Read the model definition and answer for the solid it produces. Units are mm, in the model's axes. A direction names the side the tool comes from. Give positions to 0.01 mm unless a question says otherwise; leave off trailing zeros. Order: outer loops, then holes, each group sorted by start corner. A loop starts at its lowest first (then second) coordinate and runs counter-clockwise, first axis right, second up. Notation, with made-up numbers: (14, 55) - (68, 55) arc R33 ccw to (68, 89) - close; hole circle Ø7 at (12.5, 44.5). An arc over 180 degrees is marked (long way). Use a Markdown table: item, result. Add a question column.
1. Which of the six approach directions +Z, -Z, +X, -X, +Y, -Y give full straight-line access (tool end or side, diameter ignored) to faces 4 (the cylindrical face through (-3.233, 1.341, 5.507)), 5 (the cylindrical face through (0.867, 3.905, 2.028)), 6 (the flat face through (0, -3, 5))?
2. For a pull along Z with two mould halves and no side action, classify faces 1 (the flat face through (0, 0, 12)), 2 (the cylindrical face through (1.5, -0.07, 9.04)), 3 (the flat face through (-3, 0, 4)) as released by +Z, released by -Z, zero draft, split by the parting line, or undercut.
3. A cutting plane is placed at C-C on y = -3.25. Determine the outline of the cut face in (x, z), and give its area (3 significant figures).
4. Consider L1, parallel to Z at x = 3.25, y = -0.5; L2, parallel to X at y = 0, z = 10.5; L3, parallel to Z at x = -2, y = 0.25. Determine where each line is inside the solid, lowest interval first.
5. A cutting plane is placed at D-D on z = 2.25. Determine the outline of the cut face in (x, y).
6. A cutting plane is placed at A-A on y = 0. Determine the outline of the cut face in (x, z).
7. Flat-ended cylindrical pins translate along their axes: P1, Ø1, axis at y = 1, z = 8.5, coming from the +X side; P2, Ø2, axis at x = -2.5, z = 6, coming from the +Y side. Find the tip coordinate at first contact, or state that the pin passes through.
Autodesk Inventor part; units mm, degrees
ref_plane "YZ Plane" through (0, 0, 0) normal (1, 0, 0) x (0, 1, 0)
ref_plane "XZ Plane" through (0, 0, 0) normal (0, 1, 0) x (-1, 0, 0)
ref_plane "XY Plane" through (0, 0, 0) normal (0, 0, 1) x (1, 0, 0)
sketch "スケッチ1" plane through (0, 0, 0) normal (0, 1, 0) x (-1, 0, 0)
  line L0 (0, 0) -> (0, 12)
  line L1 (0, 0) -> (4, 0)
  line L2 (4, 0) -> (4, 4)
  line L3 (4, 4) -> (2.6, 4)
  line L4 (2.6, 4) -> (2.6, 5) construction
  line L5 (2.6, 5) -> (3.5, 5)
  line L6 (3.5, 5) -> (3.5, 6)
  line L7 (3.5, 6) -> (1.5, 6)
  line L8 (1.5, 6) -> (1.5, 12)
  line L9 (1.5, 12) -> (0, 12)
  arc A0 (2.6, 5) -> (2.6, 4) centre (2.6, 4.5) ccw
  line L10 (2.6, 4.5) -> (2.1, 4.5) construction
  dimension "d4" = 1
  dimension "d5" = 6
  dimension "d7" = 4
  dimension "d8" = 6
  dimension "d11" = 2.1
  dimension "d12" = 3
  dimension "d13" = 8
  dimension "d14" = 7
revolve "回転1" add sketch "スケッチ1" angle 360 about axis through (0, 0, 0) along (0, 0, 1)
thread "ねじ1"
properties part number "SPNFL-BRN-M3-6" material "ステンレス鋼 AISI 304"
Output values:
| question | item | result |
|---|---|---|
| 1 | face 4 | +Z |
| 1 | face 5 | +Z, -Z |
| 1 | face 6 | none |
| 2 | face 1 | released by +Z |
| 2 | face 2 | zero draft |
| 2 | face 3 | undercut |
| 3 | outline | (-2.33, 0) - (2.33, 0) - (2.33, 4) - (-2.33, 4) - close; (-1.3, 5) - (1.3, 5) - (1.3, 6) - (-1.3, 6) - close |
| 3 | area | 21.3 mm² |
| 4 | L1 | 0 to 4, 5 to 6 |
| 4 | L2 | -1.5 to 1.5 |
| 4 | L3 | 0 to 6 |
| 5 | outline | circle Ø8 at (0, 0) |
| 6 | outline | (-4, 0) - (4, 0) - (4, 4) - (2.6, 4) arc R0.5 cw to (2.6, 5) - (3.5, 5) - (3.5, 6) - (1.5, 6) - (1.5, 12) - (-1.5, 12) - (-1.5, 6) - (-3.5, 6) - (-3.5, 5) - (-2.6, 5) arc R0.5 cw to (-2.6, 4) - (-4, 4) - close |
| 7 | P1 | x = 1.41 |
| 7 | P2 | y = 3.16 |
